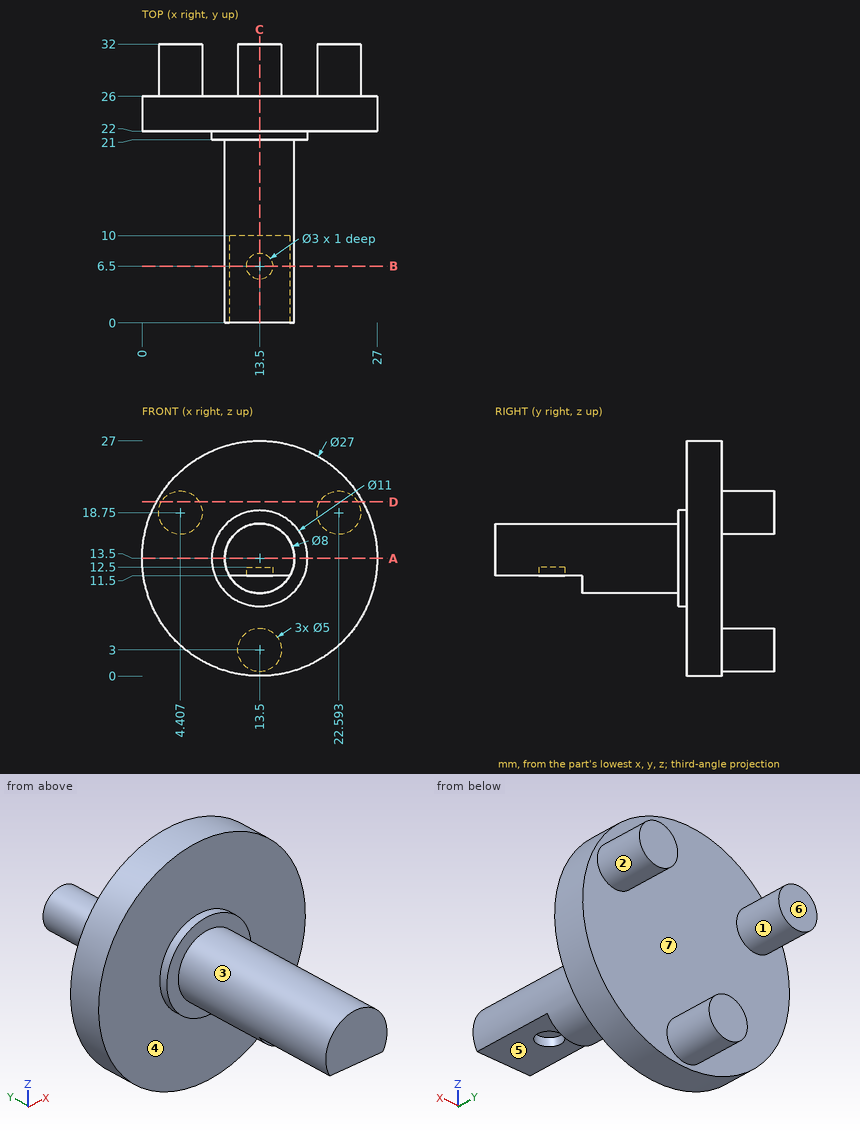
Verification items for this drawing (mm, ordinates from the low corner). A direction names the side the tool comes from. Give positions to 0.01 mm unless a question says otherwise; leave off trailing zeros. Loops run counter-clockwise (first coordinate to the right, second up) from the corner with the lowest first, then second, coordinate; pieces in that order, holes last. Notation, with made-up numbers: M 32.5,-3 L 52.5,-3 A20 ccw 52.5,27 Z; hole C -25.75,54.25 d2. An arc over 180 degrees is marked long. Write item = value, one per line. Start each with the question number.
1. Section check B-B, the plane y = 6.5. Enter the section's corners in (x, z).
2. Section check C-C, the plane x = 13.5. Enter the section's corners in (y, z).
3. Go/stop test with flat-tipped pins: P1, Ø12, axis at y = 26, z = 14, coming from the -X side; P2, Ø8, axis at x = 5.5, z = 11, coming from the +Y side; P3, Ø10, axis at x = 7, y = 25, coming from the +Z side; P4, Ø0.9, axis at x = 13.5, y = 6, coming from the -Z side. Record where each tip stops, or that it passes through.
4. Section check A-A, the plane z = 13.5. Enter the section's corners in (x, y), plus the area to 3 significant figures.
5. Thickness scan on probe 1 along Y at (x, z) = (13.5, 11.85); probe 2 along X at (y, z) = (26.5, 18); probe 3 along Y at (x, z) = (17, 17.5). Record the ranges inside material, lowest first.
6. Tool access check on the marked faces 5, 6 and 7. Record the directions out of +Z, -Z, +X, -X, +Y, -Y that give a thin tool (end or side, any length) a straight path to the whole face; none if there is none.
7. Draft check along X on the marked faces 1, 2, 3 and 4. Enter one of: +X half, -X half, draft (parallel to the pull), parting line (faces both ways), or undercut.
8. Section check D-D, the plane z = 20. Enter the section's corners in (x, y), plus the area to 3 significant figures.
Values follow:
q1.outline = M 10.04,11.5 L 12,11.5 L 12,12.5 L 15,12.5 L 15,11.5 L 16.96,11.5 A4 ccw long Z
q2.outline = M 0,11.5 L 5,11.5 L 5,12.5 L 8,12.5 L 8,11.5 L 10,11.5 L 10,9.5 L 21,9.5 L 21,8 L 22,8 L 22,0 L 26,0 L 26,0.5 L 32,0.5 L 32,5.5 L 26,5.5 L 26,27 L 22,27 L 22,19 L 21,19 L 21,17.5 L 0,17.5 Z
q3.P1 = 0
q3.P2 = 26
q3.P3 = 26.92
q3.P4 = 12.5
q4.outline = M 0,22 L 8,22 L 8,21 L 9.5,21 L 9.5,0 L 17.5,0 L 17.5,21 L 19,21 L 19,22 L 27,22 L 27,26 L 0,26 Z
q4.area = 287 mm^2
q5.probe_1 = 0 to 5, 8 to 26
q5.probe_2 = 2.02 to 6.79, 20.21 to 24.98
q5.probe_3 = 21 to 26
q6.face_5 = -Z, +X, -X, -Y
q6.face_6 = +Z, -Z, +X, -X, +Y
q6.face_7 = +Y
q7.face_1 = undercut
q7.face_2 = undercut
q7.face_3 = parting line
q7.face_4 = draft
q8.outline = M 1.67,22 L 25.33,22 L 25.33,26 L 24.76,26 L 24.76,32 L 20.43,32 L 20.43,26 L 6.57,26 L 6.57,32 L 2.24,32 L 2.24,26 L 1.67,26 Z
q8.area = 147 mm^2
